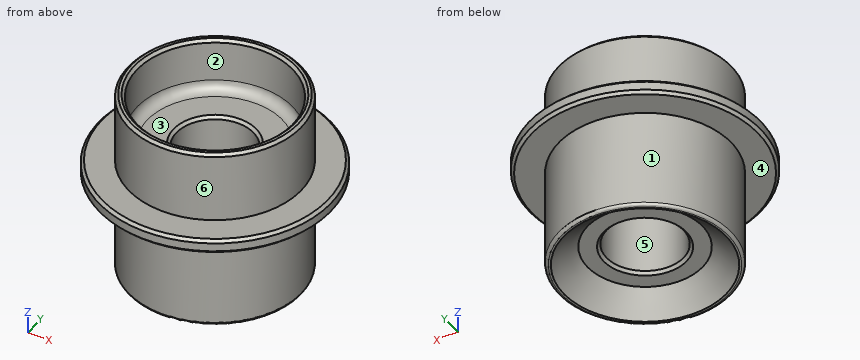
```python
from build123d import *

# Parameters (mm, degrees)
F2_R    = 0.127
F3_SIZE = 0.127
F4_SIZE = 0.127


with BuildPart() as f1:
    # F0 (on Front) → F1 (revolve)
    with BuildSketch(Plane.XZ):
        with BuildLine():
            Line((3.8608, 8.255), (3.4798, 8.255))
            Line((3.4798, 8.255), (3.4798, 6.324395))
            ThreePointArc((3.4798, 6.324395), (3.345949, 6.001251), (3.022805, 5.8674))
            Line((3.022805, 5.8674), (1.7272, 5.8674))
            Line((1.7272, 5.8674), (1.7272, 0.889))
            Line((1.7272, 0.889), (2.5781, 0.889))
            Line((2.5781, 0.889), (3.637569, 0))
            Line((3.637569, 0), (3.8608, 0))
            Line((3.8608, 0), (3.8608, 4.445))
            Line((3.8608, 4.445), (5.1816, 4.445))
            Line((5.1816, 4.445), (5.1816, 5.08))
            Line((5.1816, 5.08), (3.8608, 5.08))
            Line((3.8608, 5.08), (3.8608, 8.255))
        make_face()
    revolve(axis=Axis((0, 0, 7.74301), (0, 0, 1)))

    # F2
    f2_edges = [f1.edges().sort_by_distance(p)[0] for p in [
        (-3.8608, 0, 0),
    ]]
    fillet(f2_edges, radius=F2_R)

    # F3
    f3_edges = [f1.edges().sort_by_distance(p)[0] for p in [
        (-1.7272, 0, 0.889),
    ]]
    chamfer(f3_edges, length=F3_SIZE)

    # F4
    f4_edges = [f1.edges().sort_by_distance(p)[0] for p in [
        (-1.7272, 0, 5.8674),
        (-3.4798, 0, 8.255),
        (-3.8608, 0, 8.255),
        (-5.1816, 0, 5.08),
        (-5.1816, 0, 4.445),
    ]]
    chamfer(f4_edges, length=F4_SIZE)


solid = f1.part
```
For this review, take the finished solid that the model builds, in its own axes (mm). Face numbers are marked on the shaded views. A direction names the side the tool comes from. Give positions to 0.01 mm unless a question says otherwise; leave off trailing zeros. Order: outer loops, then holes, each group sorted by start corner. A loop starts at its lowest first (then second) coordinate and runs counter-clockwise, first axis right, second up.
1) Wall thickness on line 1 (Y direction, x = 0, z = 3.65); line 2 (Y direction, x = 0, z = 7.2); line 3 (Z direction, x = 0, y = 2): over which ranges is each line inside the solid? List them lowest first.
2) Insertion check: pin 1 (1.8 mm diameter, centred on x = -0.5, y = 0, fed in from +Z); pin 2 (3 mm diameter, centred on x = -1.5, y = -1, fed in from +Z); pin 3 (2.5 mm diameter, centred on x = -1, y = 0.5, fed in from -Z); pin 4 (2 mm diameter, centred on y = -4, z = 2.5, fed in from -X). Each pin has a flat end and moves straight along its axis. Give the tip position at first contact, or say it passes through.
3) Take a section at B-B (z = 2). Give the boundary of the cut face in (x, y), then the cut area to 3 significant figures.
4) Take a section at A-A (z = 6.5). Give the boundary of the cut face in (x, y), then the cut area to 3 significant figures.
5) The part is to be moulded in two halves that separate along Y. For the marked faces 3, 4, 5 and 6, say which applies: released by +Y, released by -Y, zero draft, split by the parting line, or undercut.
6) For the marked faces 1 and 2, list the 3-axis set-ups (+Z, -Z, +X, -X, +Y, -Y) from which the entire face can be reached by the end or side of a thin tool; tool diameter is ignored.
Derived:
1. line 1: y = -3.86 to -1.73, 1.73 to 3.86
1. line 2: y = -3.86 to -3.48, 3.48 to 3.86
1. line 3: z = 0.89 to 5.87
2. pin 1: passes through
2. pin 2: stops at z = 5.96
2. pin 3: stops at z = 0.89
2. pin 4: stops at x = -2.43
3. outline: circle Ø7.72 at (0, 0); hole circle Ø3.45 at (0, 0)
3. area: 37.5 mm2
4. outline: circle Ø7.72 at (0, 0); hole circle Ø6.96 at (0, 0)
4. area: 8.79 mm2
5. face 3: undercut
5. face 4: zero draft
5. face 5: undercut
5. face 6: split by the parting line
6. face 1: -Z
6. face 2: +Z
